Input: part model. Units: mm. Frame: model coordinates. A direction names the side the tool comes from. Round coordinates to 2 decimals unless told otherwise and drop trailing zeros. Loops run counter-clockwise (first coordinate to the right, second up) from the corner with the lowest first, then second, coordinate; pieces in that order, holes last.
(1) Draft query along Y for faces 6 (the face through (12, 24.823, 0)), 7 (the face through (3, 31, 0)), 8 (the face through (20.767, 48.528, 4.437)). Return one class per face: released by +Y, released by -Y, zero draft, split by the parting line, or undercut.
(2) Cut plane B-B, the plane x = 28. Output: boundary loops of the cut face in (y, z).
(3) First-contact query: pin 1 Ø1 at (x, z) = (9.5, 3) entering from +Y; pin 2 Ø1 at (y, z) = (29.5, 5) entering from +X; pin 3 Ø5 at (y, z) = (28, 2) entering from -X (3 decimals); pin 4 Ø13 at (x, y) = (22.54, 56.53) entering from -Z. Flat tips, straight axial feed; report the tip coordinate or a pass-through.
(4) Line query: line 1 (Y direction, x = 3.5, z = 3.5); line 2 (Y direction, x = 19, z = -2.5); line 3 (X direction, y = 57, z = 1.5). Output: solid intervals per line, ascending.
(5) Cut plane A-A, the plane y = 29.5. Output: boundary loops of the cut face in (x, z).
(6) Cut plane C-C, the plane x = 7.5. Output: boundary loops of the cut face in (y, z).
(7) Cut plane D-D, the plane z = 8.25. Output: boundary loops of the cut face in (x, y), and give its area (3 significant figures).
(8) Access query for faces 1 (the face through (0.295, 27, 3)), 2 (the face through (22, 45, 0)), 3 (the face through (25.044, 36, 5)), 4 (the face through (15.07, 25.76, 2.04)), 5 (the face through (20.044, 38, 4)). Directions: +Z, -Z, +X, -X, +Y, -Y. A direction counts if a zero-diameter tool reaches every point of the face in a straight line with its end or side. Return the directions, or none.
from build123d import *

# Parameters (mm, degrees)
SKETCH1_R             = 9.2
SKETCH1_R_2           = 8.2
BOSS_EXTRUDE1_DEPTH   = 9
BOSS_EXTRUDE1_2_DEPTH = 9
BOSS_EXTRUDE2_DEPTH   = 9
SKETCH3_W             = 24.749470463
SKETCH3_H             = 15
BOSS_EXTRUDE3_DEPTH   = 3


with BuildPart() as part:
    # Sketch1 → Boss-Extrude1 (new body)
    with BuildSketch(Plane.XY):
        with Locations((22.544450453, 56.532786317)):
            Circle(SKETCH1_R)
        with Locations((22.544450453, 56.532786317)):
            Circle(SKETCH1_R_2, mode=Mode.SUBTRACT)
    extrude(amount=BOSS_EXTRUDE1_DEPTH)



with BuildPart() as body_2:
    # Sketch1 → Boss-Extrude1 2 (new body)
    with BuildSketch(Plane.XY):
        with Locations((2.62521603, 39.822786317)):
            Circle(SKETCH1_R)
        with Locations((2.62521603, 39.822786317)):
            Circle(SKETCH1_R_2, mode=Mode.SUBTRACT)
    extrude(amount=BOSS_EXTRUDE1_2_DEPTH)


with BuildPart() as part_1:
    add(part.part)

    add(body_2.part)  # Boss-Extrude2 merges body 2
    # Sketch2 → Boss-Extrude2 (add)
    with BuildSketch(Plane.XY):
        with BuildLine():
            Line((0.29497999, 24.822786317), (5.29497999, 24.822786317))
            Line((5.29497999, 24.822786317), (5.29497999, 31.018675891))
            ThreePointArc((5.29497999, 31.018675891), (2.801620408, 30.624477696), (0.29497999, 30.922786317))
            Line((0.29497999, 30.922786317), (0.29497999, 24.822786317))
        make_face()
        with BuildLine():
            Line((20.044450453, 47.722786317), (20.044450453, 24.822786317))
            Line((20.044450453, 24.822786317), (25.044450453, 24.822786317))
            Line((25.044450453, 24.822786317), (25.044450453, 47.722786317))
            ThreePointArc((25.044450453, 47.722786317), (22.544450453, 47.332786317), (20.044450453, 47.722786317))
        make_face()
    extrude(amount=BOSS_EXTRUDE2_DEPTH)

    # Sketch3 → Boss-Extrude3 (add)
    with BuildSketch(Plane.XZ.offset(-24.822786317)):
        with Locations((12.669715222, 1.5)):
            Rectangle(SKETCH3_W, SKETCH3_H)
    extrude(amount=-BOSS_EXTRUDE3_DEPTH)

    # Sketch5 → Avellanado para tornillo con cabeza avellanada en cruz de M31 (revolve, cut)
    with BuildSketch(Plane(origin=(13.312105777, 27.822786317, 2.425807985), x_dir=(0, 0, 1), z_dir=(1, 0, 0))):
        Polygon((0, 0), (0, 11.081549114), (1.8, 10), (1.8, 1.15882653), (3, 0), align=None)
    revolve(axis=Axis((13.312105777, 34.172786317, 2.425807985), (0, -1, 0)), mode=Mode.SUBTRACT)


solid = part_1.part
Reported:
1. face 6: released by -Y
1. face 7: zero draft
1. face 8: undercut
2. outline: (49.12, 0) - (50.41, 0) - (50.41, 9) - (49.12, 9) - close; (62.65, 0) - (63.94, 0) - (63.94, 9) - (62.65, 9) - close
3. pin 1: stops at y = 46.46
3. pin 2: stops at x = 25.04
3. pin 3: stops at x = 0.295
3. pin 4: passes through
4. line 1: y = 24.82 to 31.67, 47.98 to 48.98
4. line 2: y = 24.82 to 27.82
4. line 3: x = 13.36 to 14.36, 30.73 to 31.73
5. outline: (0.29, 0) - (5.29, 0) - (5.29, 9) - (0.29, 9) - close; (20.04, 0) - (25.04, 0) - (25.04, 9) - (20.04, 9) - close
6. outline: (24.82, -6) - (27.82, -6) - (27.82, 9) - (24.82, 9) - close; (32.02, 0) - (33.23, 0) - (33.23, 9) - (32.02, 9) - close; (46.42, 0) - (47.63, 0) - (47.63, 9) - (46.42, 9) - close
7. outline: (0.29, 24.82) - (25.04, 24.82) - (25.04, 47.68) arc R9.2 ccw (long way) to (20.04, 47.68) - (20.04, 27.82) - (5.29, 27.82) - (5.29, 31.02) arc R9.2 ccw (long way) to (0.29, 30.92) - close; hole circle Ø16.4 at (2.63, 39.82); hole circle Ø16.4 at (22.54, 56.53)
7. area: 296 mm2
8. face 1: +Z, -Z, -X, -Y
8. face 2: -Z, +X, -X, +Y
8. face 3: +Z, -Z, +X, -Y
8. face 4: -Y
8. face 5: +Z, -Z
